CAD build for the part. Positions are in the model's coordinates, mm. Face numbers are marked on the shaded views. Round coordinates to 2 decimals unless told otherwise and drop trailing zeros. Order: outer loops, then holes, each group sorted by start corner. A loop starts at its lowest first (then second) coordinate and runs counter-clockwise, first axis right, second up. Notation, with made-up numbers: M 32.5,62.25 L 46.5,62.25 A15 cw 46.5,80.25 Z; hole C -2.5,-31 d9. An arc over 180 degrees is marked long. Answer as a JSON object with one key per item and string values.
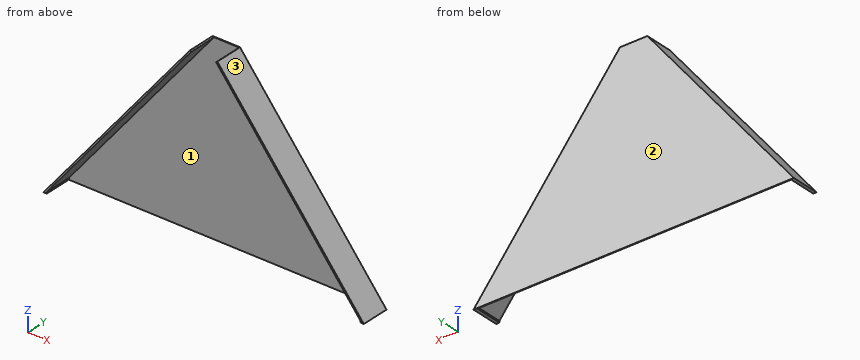
```python
from build123d import *

# Parameters (mm, degrees)
BOSS_EXTRUDE1_DEPTH     = 35
CUT_EXTRUDE1_DEPTH      = 314.199217751
CUT_EXTRUDE1_DEPTH_BACK = 314.199217751
SKETCH2_W               = 401.672921909
SKETCH2_H               = 2
BOSS_EXTRUDE2_DEPTH     = 1


with BuildPart() as part:
    # Sketch1 → Boss-Extrude1 (new body)
    with BuildSketch(Plane(origin=(0, 0, 0), x_dir=(1, 0, 0), z_dir=(0, 1, 0))):
        Polygon((-205, 0), (205, 0), (17.5, -234.18742494), (15.9387505, -232.93742494), (200.836668001, -2), (-200.836668001, -2), (-15.9387505, -232.93742494), (-17.5, -234.18742494), align=None)
    extrude(amount=BOSS_EXTRUDE1_DEPTH)

    # Sketch2 → Cut-Extrude1 (cut, two sides: drawn at the far end of the back side and taken through both)
    with BuildSketch(Plane(origin=(0, 35, 0), x_dir=(1, 0, 0), z_dir=(0, 1, 0)).offset(-CUT_EXTRUDE1_DEPTH_BACK)):
        with Locations((-0.000207047, -1)):
            Rectangle(SKETCH2_W, SKETCH2_H)
    extrude(amount=CUT_EXTRUDE1_DEPTH + CUT_EXTRUDE1_DEPTH_BACK, mode=Mode.SUBTRACT)


with BuildPart() as cut_extrude1_piece_1:
    # of the separate pieces the step leaves, piece 1, a body of its own (cut_extrude1_pieces)
    add(part.part.solids().sort_by_distance((200.836253908, 0, 0))[0])



with BuildPart() as cut_extrude1_piece_2:
    # of the separate pieces the step leaves, piece 2, a body of its own (cut_extrude1_pieces)
    add(part.part.solids().sort_by_distance((-205, 0, 0))[0])


with BuildPart() as cut_extrude1_piece_1_1:
    add(cut_extrude1_piece_1.part)

    add(cut_extrude1_piece_2.part)  # Boss-Extrude2 merges Cut-Extrude1 piece 2
    # Sketch3 → Boss-Extrude2 (add)
    with BuildSketch(Plane(origin=(0, 35, 0), x_dir=(1, 0, 0), z_dir=(0, 1, 0))):
        Polygon((-205, 0), (-17.5, -234.18742494), (17.5, -234.18742494), (205, 0), align=None)
    extrude(amount=BOSS_EXTRUDE2_DEPTH)


solid = cut_extrude1_piece_1_1.part
```
Item 1: Drop flat-ended pins along their axis: pin 1 Ø1.5 at (x, y) = (-14, 14.5) entering from -Z; pin 2 Ø2 at (y, z) = (22.5, 30) entering from -X; pin 3 Ø1.5 at (x, y) = (-30.5, 8.5) entering from +Z; pin 4 Ø6 at (y, z) = (22, 186) entering from +X. Give the stop position or say it passes through.
Worked answers:
{"pin 1": "passes through", "pin 2": "stops at x = -181.78", "pin 3": "stops at z = 218.89", "pin 4": "stops at x = 58.48"}
Item 2: Saw through at B-B on z = 152.5. List the corners of the cut face in (x, y), and give its area (3 significant figures).
Worked answers:
{"outline": "M -82.9,0 L -80.34,0 L -80.34,35 L 80.34,35 L 80.34,0 L 82.9,0 L 82.9,36 L -82.9,36 Z", "area": "345 mm2"}
Item 3: Saw through at D-D on z = 177.5. List the corners of the cut face in (x, y).
Worked answers:
{"outline": "M -62.89,0 L -60.32,0 L -60.32,35 L 60.32,35 L 60.32,0 L 62.89,0 L 62.89,36 L -62.89,36 Z"}
Item 4: Wall check: line 1 along Y through (x, z) = (136, 50); line 2 along X through (y, z) = (30.5, 119); line 3 along X through (y, z) = (32, 25.5). Give the ranges that are in metal, low to high. Write a range as [from, to].
Worked answers:
{"line 1": "y = [35, 36]", "line 2": "x = [-109.72, -107.16], [107.16, 109.72]", "line 3": "x = [-184.58, -182.02], [182.02, 184.58]"}
Item 5: Two-plate mould, pull along X, no slides. Class the marked faces 1, 2 and 3: released by +X, released by -X, zero draft, split by the parting line, or undercut.
Worked answers:
{"face 1": "undercut", "face 2": "zero draft", "face 3": "released by +X"}
Item 6: Saw through at C-C on x = -7.5. List the corners of the cut face in (y, z).
Worked answers:
{"outline": "M 35,0 L 36,0 L 36,234.19 L 35,234.19 Z"}
